from build123d import *

# Parameters (mm, degrees)
F1_DEPTH = 5
F2_R     = 1.5
F3_DEPTH = 25.4


with BuildPart() as f1:
    # F0 (on Top) → F1 (new body)
    with BuildSketch(Plane.XY):
        with BuildLine():
            Line((-10.2344341576, 0.7447922041), (-4.9204421579, 0.7447922041))
            ThreePointArc((-4.9204421579, 0.7447922041), (-4.6921521255, 1.6580635959), (-4.2959631379, 2.5120046127))
            Line((-4.2959631379, 2.5120046127), (-10.2344341576, 2.5120046127))
            Line((-10.2344341576, 2.5120046127), (-10.2344341576, 0.7447922041))
        make_face()
        with BuildLine():
            ThreePointArc((-4.2756532365, -2.5464202045), (-4.6795608737, -1.6932738958), (-4.9151095275, -0.7792077959))
            Line((-4.9151095275, -0.7792077959), (-10.2344341576, -0.7792077959))
            Line((-10.2344341576, -0.7792077959), (-10.2344341576, -2.5464202045))
            Line((-10.2344341576, -2.5464202045), (-4.2756532365, -2.5464202045))
        make_face()
        with BuildLine():
            ThreePointArc((-3.9061193363, 0.7447922041), (0.3740546925, 3.9588592781), (3.9764913802, 0))
            ThreePointArc((3.9764913802, 0), (0.391506034, -3.9571715558), (-3.8993998137, -0.7792077959))
            Line((-3.8993998137, -0.7792077959), (-4.9151095275, -0.7792077959))
            ThreePointArc((-4.9151095275, -0.7792077959), (-4.6795608737, -1.6932738958), (-4.2756532365, -2.5464202045))
            ThreePointArc((-4.2756532365, -2.5464202045), (1.3205519643, -4.7980838849), (4.9764913802, 0))
            ThreePointArc((4.9764913802, 0), (1.3012768598, 4.8033472695), (-4.2959631379, 2.5120046127))
            ThreePointArc((-4.2959631379, 2.5120046127), (-4.6921521255, 1.6580635959), (-4.9204421579, 0.7447922041))
            Line((-4.9204421579, 0.7447922041), (-3.9061193363, 0.7447922041))
        make_face()
    extrude(amount=F1_DEPTH)

    # F2 (on face) → F3 (cut)
    with BuildSketch(Plane.XZ.offset(2.5464202045)):
        with Locations((-7.4309720658, 2.4591526017)):
            Circle(F2_R)
    extrude(amount=-F3_DEPTH, mode=Mode.SUBTRACT)


solid = f1.part
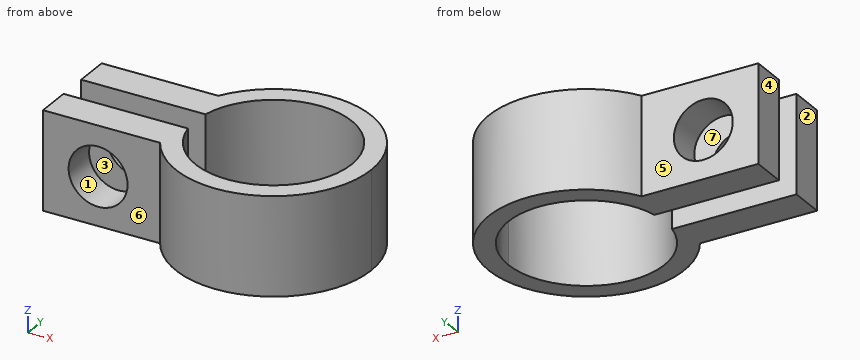
Geometry: final body of the model. Coordinates: model frame, mm. Face numbers are marked on the shaded views. A direction names the side the tool comes from. Give positions to 0.01 mm unless a question says otherwise; leave off trailing zeros. Write each loop counter-clockwise with the first axis right and the second up, starting at its lowest first coordinate (ties: lowest second). Pieces come first, ordered by that corner, then holes.
(1) Cut plane D-D, the plane y = -3.5. Return loops of the section in (x, z).
(2) Cut plane A-A, the plane x = -5. Return loops of the section in (y, z), then the cut area to 3 significant figures.
(3) Ray query, line 1 (X direction, y = 1, z = 1.7); line 2 (Y direction, x = -5.5, z = 3.7); line 3 (Y direction, x = 1.25, z = 3.9). Return the intervals inside material, ascending.
(4) First-contact query: P1, Ø1, axis at x = -5, z = 4.5, coming from the -Y side; P2, Ø2.5, axis at x = -8.5, z = 1.5, coming from the +Y side; P3, Ø1.5, axis at x = -5, y = 0.5, coming from the +Z side. Flat tips, straight axial feed; report the tip coordinate or a pass-through.
(5) Cut plane B-B, the plane z = 1.85. Return loops of the section in (x, y).
(6) Access query for the marked faces 4, 5, 6 and 7. Directions: +Z, -Z, +X, -X, +Y, -Y. A direction counts if a zero-diameter tool reaches every point of the face in a straight line with its end or side. Return the directions, or none.
(7) Cut plane C-C, the plane y = -2. Return loops of the section in (x, z), then the cut area to 3 significant figures.
(8) Mould query, pull axis X, two halves, no side actions, for the marked faces 1, 2 and 3. Classes: released by +X, released by -X, zero draft, split by the parting line, or undercut.
Values follow:
1. outline: (-3.54, 0) - (-1.89, 0) - (-1.89, 5) - (-3.54, 5) - close; (1.89, 0) - (3.54, 0) - (3.54, 5) - (1.89, 5) - close
2. outline: (-2.55, 0) - (-0.78, 0) - (-0.78, 5) - (-2.55, 5) - close; (0.74, 0) - (2.51, 0) - (2.51, 5) - (0.74, 5) - close
2. area: 17.7 mm2
3. line 1: x = -10.23 to -8.72, -6.14 to -3.85, 3.85 to 4.87
3. line 2: y = -2.55 to -0.78, 0.74 to 2.51
3. line 3: y = -4.82 to -3.77, 3.77 to 4.82
4. P1: stops at y = -2.55
4. P2: stops at y = 2.51
4. P3: stops at z = 5
5. outline: (-10.23, -2.55) - (-8.8, -2.55) - (-8.8, -0.78) - (-10.23, -0.78) - close; (-10.23, 0.74) - (-8.8, 0.74) - (-8.8, 2.51) - (-10.23, 2.51) - close; (-6.06, -2.55) - (-4.28, -2.55) arc R4.98 ccw (long way) to (-4.3, 2.51) - (-6.06, 2.51) - (-6.06, 0.74) - (-3.91, 0.74) arc R3.98 cw (long way) to (-3.9, -0.78) - (-6.06, -0.78) - close
6. face 4: +Z, -Z, -X, +Y, -Y
6. face 5: +Z, -Z, -X, +Y
6. face 6: +Z, -Z, -X, -Y
6. face 7: +Z, -Z, -X
7. outline: (-10.23, 0) - (-3.44, 0) - (-3.44, 5) - (-10.23, 5) - close; (3.44, 0) - (4.56, 0) - (4.56, 5) - (3.44, 5) - close; hole circle Ø3 at (-7.43, 2.46)
7. area: 32.5 mm2
8. face 1: undercut
8. face 2: released by -X
8. face 3: zero draft
